Design review of the part shown in the three views and the two pictorial views. Dimensions are in mm from the part's minimum x, y and z. A direction names the side the tool comes from. Round coordinates to 2 decimals unless told otherwise and drop trailing zeros. Loops run counter-clockwise (first coordinate to the right, second up) from the corner with the lowest first, then second, coordinate; pieces in that order, holes last. Notation, with made-up numbers: M 80,-24.5 L 105,-24.5 A21 cw 105,-5.5 Z; hole C -24,-13.5 d11. An arc over 180 degrees is marked long. Return JSON: item names as keys, results as strings. Group by question number.
Q1. Consider section A-A (x = 17). State the section outline as (y, z) points.
Q2. Consider section B-B (y = 6.5). State the section outline as (x, z) points.
Q3. Draft analysis for pull direction Y (two halves, no side actions). For the marked faces 5, 6 and 7, state which applies: pulls with the +Y half, pulls with the -Y half, needs draft (parallel to the pull), parting line crosses it, or undercut.
Q4. To check wall thickness, follow line 1 along Z through (x, y) = (9, 10.5); line 2 along Z through (x, y) = (19, 15); line 3 along X through (y, z) = (2.5, 3). State the ranges of each line that lie inside material, in increasing order.
Q5. For the marked faces 1, 2, 3 and 4, list the 3-axis set-ups (+Z, -Z, +X, -X, +Y, -Y) from which the entire face can be reached by the end or side of a thin tool; tool diameter is ignored.
Q6. Consider section C-C (z = 29). State the section outline as (x, y) points.
Q7. Clearance check with flat-ended pins moving along their axes: pin 1 Ø5 at (x, y) = (15.5, 7) entering from +Z; pin 2 Ø4 at (x, z) = (35, 27.5) entering from +Y; pin 3 Ø8 at (y, z) = (15, 32) entering from +X. State where each tip first meets the part, or that it passes through.
Q8. Consider section D-D (y = 22.5). State the section outline as (x, z) points, and give its area (3 significant figures).
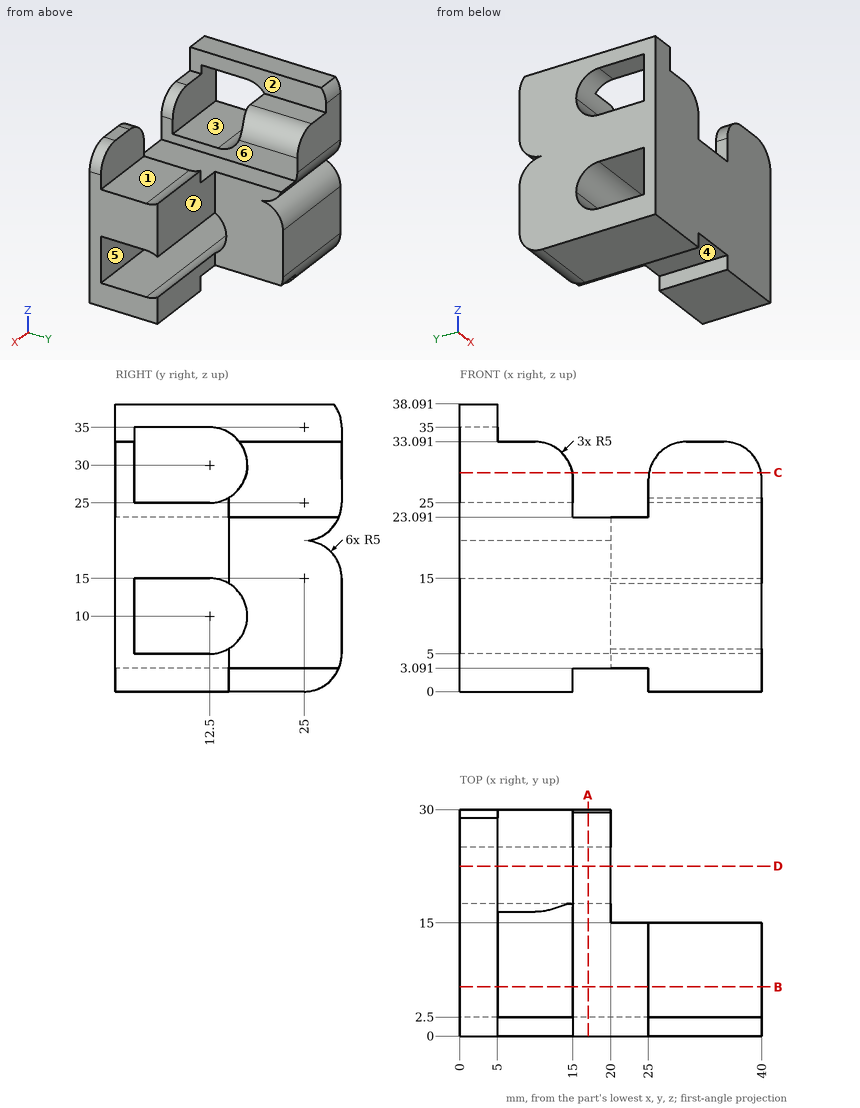
Values:
{
 "1": {"outline": "M 0,3.09 L 29.62,3.09 A5 ccw 30,5 L 30,15 A5 ccw 25,20 A5 ccw 29.62,23.09 L 0,23.09 Z; hole M 2.5,5 L 12.5,5 A5 ccw 12.5,15 L 2.5,15 Z"},
 "2": {"outline": "M 0,0 L 15,0 L 15,3.09 L 25,3.09 L 25,0 L 40,0 L 40,5 L 0,5 Z; M 0,15 L 40,15 L 40,25 L 25,25 L 25,23.09 L 15,23.09 L 15,25 L 0,25 Z; M 0,35 L 5,35 L 5,38.09 L 0,38.09 Z"},
 "3": {"face 5": "undercut", "face 6": "needs draft", "face 7": "pulls with the +Y half"},
 "4": {"line 1": "z = 0 to 5, 15 to 25", "line 2": "z = 3.09 to 5.67, 14.33 to 23.09", "line 3": "x = 0 to 15, 25 to 40"},
 "5": {"face 1": "+Z, +X, -X", "face 2": "+Z, +X, +Y, -Y", "face 3": "+X, -X", "face 4": "-Z, +Y, -Y"},
 "6": {"outline": "M 0,0 L 14.92,0 L 14.92,2.5 L 0,2.5 Z; M 0,17.4 L 14.92,17.4 L 14.92,30 L 0,30 Z; M 25.08,0 L 39.92,0 L 39.92,2.5 L 25.08,2.5 Z"},
 "7": {"pin 1": "stops at z = 25", "pin 2": "stops at y = 15", "pin 3": "stops at x = 14.96"},
 "8": {"outline": "M 0,0 L 15,0 L 15,3.09 L 20,3.09 L 20,23.09 L 15,23.09 L 15,28.09 A5 ccw 10,33.09 L 5,33.09 L 5,38.09 L 0,38.09 Z", "area": "616 mm2"}
}
